For this review, take the finished solid that the model builds, in its own axes (mm). A direction names the side the tool comes from. Round coordinates to 2 decimals unless told otherwise and drop trailing zeros. Order: outer loops, then holes, each group sorted by start corner. A loop starts at its lowest first (then second) coordinate and runs counter-clockwise, first axis right, second up. Notation, with made-up numbers: (33.5, 81) - (37.5, 81) arc R26 cw to (37.5, 106) - close; hole circle Ø4 at (63, 67.5). An arc over 180 degrees is marked (long way). One line per item, written item: value.
```python
from build123d import *

# Parameters (mm, degrees)
SCHNITT_LINEAR_AUSTRAGEN1_DEPTH      = 1.2
SKIZZE3_W                            = 24
SKIZZE3_H                            = 24
SCHNITT_LINEAR_AUSTRAGEN2_DEPTH      = 6.6
AUFSATZ_LINEAR_AUSTRAGEN1_DEPTH      = 11.25
SKIZZE8_W                            = 5.9
SKIZZE8_H                            = 0.5
SCHNITT_LINEAR_AUSTRAGEN3_DEPTH      = 0.4
SCHNITT_LINEAR_AUSTRAGEN3_DEPTH_BACK = 0.4


with BuildPart() as part:
    # Skizze1 → Rotation1 (revolve)
    with BuildSketch(Plane(origin=(0, 0, 0), x_dir=(0, 0, -1), z_dir=(1, 0, 0))):
        with BuildLine():
            Line((0, 12.5), (2.1915, 12.5))
            Line((2.1915, 12.5), (3.15, 10.9))
            Line((3.15, 10.9), (3.15, 12.1))
            Line((3.15, 12.1), (3.336523063, 12.5))
            Line((3.336523063, 12.5), (3.55, 12.5))
            Line((3.55, 12.5), (3.75, 12.3))
            Line((3.75, 12.3), (3.75, 10.9))
            Line((3.75, 10.9), (5.75, 10.9))
            Line((5.75, 10.9), (6.7, 10.351517244))
            Line((6.7, 10.351517244), (6.7, 4.4))
            Line((6.7, 4.4), (6.9, 4.4))
            Line((6.9, 4.4), (6.9, -11.5))
            Line((6.9, -11.5), (6.075, -11.5))
            ThreePointArc((6.075, -11.5), (6.162867966, -11.712132034), (6.375, -11.8))
            Line((6.375, -11.8), (6.75, -11.8))
            Line((6.75, -11.8), (6.75, -12.6))
            Line((6.75, -12.6), (6.575, -12.6))
            Line((6.575, -12.6), (6.575, -14.2))
            Line((6.575, -14.2), (4.864, -14.2))
            Line((4.864, -14.2), (4.864, -18.669))
            Line((4.864, -18.669), (4.283, -19.25))
            Line((4.283, -19.25), (0, -19.25))
            Line((0, -19.25), (0, 12.5))
        make_face()
    revolve(axis=Axis((0, -19.25, 0), (0, 1, 0)))

    # Skizze2 → Schnitt-Linear austragen1 (cut)
    with BuildSketch(Plane(origin=(0, 12.5, 0), x_dir=(1, 0, 0), z_dir=(0, 1, 0))):
        with BuildLine():
            Line((-3.07408523, -0.4), (3.07408523, -0.4))
            ThreePointArc((3.07408523, -0.4), (3.1, 0), (3.07408523, 0.4))
            Line((3.07408523, 0.4), (-3.07408523, 0.4))
            ThreePointArc((-3.07408523, 0.4), (-3.1, 0), (-3.07408523, -0.4))
        make_face()
    extrude(amount=-SCHNITT_LINEAR_AUSTRAGEN1_DEPTH, mode=Mode.SUBTRACT)

    # Skizze3 → Schnitt-Linear austragen2 (cut)
    with BuildSketch(Plane(origin=(0, 12.5, 0), x_dir=(1, 0, 0), z_dir=(0, 1, 0))):
        Rectangle(SKIZZE3_W, SKIZZE3_H)
        Polygon((-6, -3.464101615), (0, -6.92820323), (6, -3.464101615), (6, 3.464101615), (0, 6.92820323), (-6, 3.464101615), align=None, mode=Mode.SUBTRACT)
    extrude(amount=-SCHNITT_LINEAR_AUSTRAGEN2_DEPTH, mode=Mode.SUBTRACT)

    # Skizze4 → Rotation2 (revolve)
    with BuildSketch(Plane(origin=(0, 0, 0), x_dir=(0, 0, -1), z_dir=(1, 0, 0))):
        with BuildLine():
            Line((-22.5, 0), (-22.5, 2.4))
            Line((-22.5, 2.4), (-22.079507824, 4.784729636))
            ThreePointArc((-22.079507824, 4.784729636), (-22.011103795, 4.903208889), (-21.882546273, 4.95))
            Line((-21.882546273, 4.95), (-21, 4.95))
            Line((-21, 4.95), (-21, 3.1))
            ThreePointArc((-21, 3.1), (-20.882842712, 2.817157288), (-20.6, 2.7))
            Line((-20.6, 2.7), (-19.875, 2.7))
            Line((-19.875, 2.7), (-19.875, 3.55))
            Line((-19.875, 3.55), (-19.675, 3.75))
            Line((-19.675, 3.75), (-18.6, 3.75))
            Line((-18.6, 3.75), (-18.6, 4.85))
            Line((-18.6, 4.85), (-17.1, 4.85))
            Line((-17.1, 4.85), (-16.666987298, 5.1))
            Line((-16.666987298, 5.1), (-9.5, 5.1))
            Line((-9.5, 5.1), (-8, 3.6))
            Line((-8, 3.6), (0, 3.6))
            Line((0, 3.6), (0, 0))
            Line((0, 0), (-22.5, 0))
        make_face()
    revolve(axis=Axis((0, 0, 0), (0, 0, 1)))

    # Skizze5 → Aufsatz-Linear austragen1 (add)
    with BuildSketch(Plane.XY):
        with BuildLine():
            Line((-3.815756806, -1.5), (3.815756806, -1.5))
            ThreePointArc((3.815756806, -1.5), (4.1, 0), (3.815756806, 1.5))
            Line((3.815756806, 1.5), (-3.815756806, 1.5))
            ThreePointArc((-3.815756806, 1.5), (-4.1, 0), (-3.815756806, -1.5))
        make_face()
    extrude(amount=AUFSATZ_LINEAR_AUSTRAGEN1_DEPTH)

    # Skizze6 → Schnitt-Rotation1 (revolve, cut)
    with BuildSketch(Plane(origin=(0, 0, 0), x_dir=(0, 0, -1), z_dir=(1, 0, 0))):
        with BuildLine():
            Line((-22.5, 0), (-22.5, 2.4))
            ThreePointArc((-22.5, 2.4), (-22.412132034, 2.187867966), (-22.2, 2.1))
            Line((-22.2, 2.1), (-7.5, 2.1))
            Line((-7.5, 2.1), (-7.5, 1.5))
            Line((-7.5, 1.5), (0, 1.5))
            Line((0, 1.5), (0, 0))
            Line((0, 0), (-22.5, 0))
        make_face()
    revolve(axis=Axis((0, 0, 0), (0, 0, 1)), mode=Mode.SUBTRACT)

    # Skizze7 → Schnitt-Rotation2 (revolve, cut)
    with BuildSketch(Plane(origin=(0, 0, 0), x_dir=(0, 0, -1), z_dir=(1, 0, 0))):
        with BuildLine():
            Line((1.5, 0.1), (1.5, -19.05))
            Line((1.5, -19.05), (1.615470054, -19.25))
            Line((1.615470054, -19.25), (0, -19.25))
            Line((0, -19.25), (0, 1.6))
            ThreePointArc((0, 1.6), (1.060660172, 1.160660172), (1.5, 0.1))
        make_face()
    revolve(axis=Axis((0, -19.25, 0), (0, 1, 0)), mode=Mode.SUBTRACT)

    # Skizze8 → Schnitt-Linear austragen3 (cut, two sides)
    with BuildSketch(Plane.XY) as schnitt_linear_austragen3_sk:
        with Locations((0, 11.25)):
            Rectangle(SKIZZE8_W, SKIZZE8_H)
    extrude(amount=SCHNITT_LINEAR_AUSTRAGEN3_DEPTH, mode=Mode.SUBTRACT)
    extrude(schnitt_linear_austragen3_sk.sketch, amount=-SCHNITT_LINEAR_AUSTRAGEN3_DEPTH_BACK, mode=Mode.SUBTRACT)


solid = part.part
```
Item 1: For P1, Ø1, axis at x = 3, y = 1, coming from the -Z side; P2, Ø0.9, axis at x = 4, z = -6, coming from the +Y side; P3, Ø1, axis at y = 4.5, z = 16.5, coming from the -X side; P4, Ø4, axis at y = -9, z = 9, coming from the +X side, all flat-tipped, find the tip position at first contact; note any pin that passes through.
Returned:
P1: z = -6.43
P2: y = 4.4
P3: x = -3.16
P4: through
Item 2: Machinability: for faces 1 (the cylindrical face through (-1.457, 4.626, 17.84)), 2 (the flat face through (2.96, 8.36, 5.22)), 3 (the cylindrical face through (-0.631, 2.003, 14.747)), which of the approach directions +Z, -Z, +X, -X, +Y, -Y give a long, thin tool a straight path to every point of the face, cutting with its end or side? Answer none if there is none.
Returned:
face 1: none
face 2: +Z, +X, +Y
face 3: +Z
Item 3: Take a section at B-B (z = 12.5). Write out the cut boundary in (x, y), plus the area to 3 significant figures.
Returned:
outline: circle Ø10.2 at (0, 0); hole circle Ø4.2 at (0, 0)
area: 67.9 mm^2
Item 4: Take a section at A-A (y = -10). Write out the cut boundary in (x, z), plus the area to 3 significant figures.
Returned:
outline: circle Ø13.8 at (0, 0); hole circle Ø3 at (0, 0)
area: 143 mm^2
Item 5: The part is to be moulded in two halves that separate along Y. For faces 4 (the cylindrical face through (0.575, 1.386, 3.698)), 5 (the flat face through (3.2, 5.9, 5.4)), 6 (the flat face through (0, 12, 0.4)), say which applies: +Y half, -Y half, draft (parallel to the pull), parting line (faces both ways), or undercut.
Returned:
face 4: undercut
face 5: +Y half
face 6: draft
Item 6: Wall thickness on line 1 (Y direction, x = 0, z = 15.25); line 2 (Z direction, x = 0, y = -13) (3 decimals); line 3 (Y direction, x = 0, z = 2): over which ranges is each line inside the solid? List them lowest first.
Returned:
line 1: -5.1 to -2.1, 2.1 to 5.1
line 2: -6.575 to -1.5, 1.5 to 6.575
line 3: -19.25 to -1.5, 1.5 to 12.5
